Work out the finished part from the listing and answer in its coordinate system (mm). Round coordinates to 2 decimals unless told otherwise and drop trailing zeros. Write each loop counter-clockwise with the first axis right and the second up, starting at its lowest first coordinate (ties: lowest second). Pieces come first, ordered by that corner, then holes. Notation, with made-up numbers: (12, 50) -> (49, 50) arc R27 cw to (49, 81) -> close; hole circle Ø1 at (78, -7.5). An arc over 180 degrees is marked (long way). One line per item, written item: value.
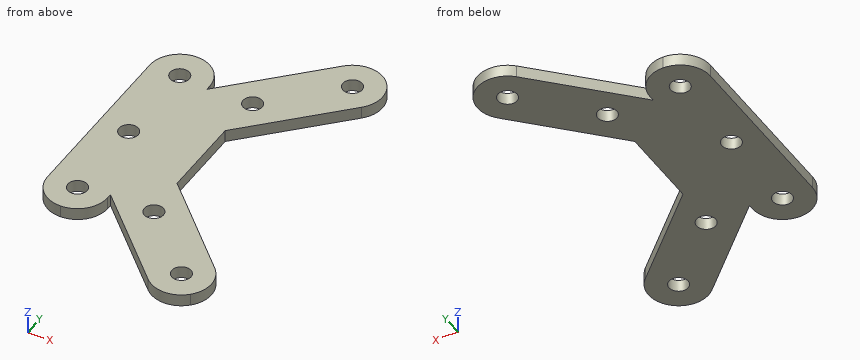
```python
from build123d import *

# Parameters (mm, degrees)
SKETCH_1_R          = 1.6
EXTRUDE_1_DEPTH     = 1
SKETCH_2_R          = 1.6
CUT_EXTRUDE_1_DEPTH = 45.10524807
FILLET_1_R          = 5


with BuildPart() as part:
    # ｽｹｯﾁ1 → ﾎﾞｽ - 押し出し1 (new, symmetric)
    with BuildSketch(Plane.XY):
        Polygon((5, 20), (-5, 20), (-5, -20), (5, -20), (5, -14.142135624), (23.03122292, -32.173358544), (30.102290732, -25.102290732), (12.071067812, -7.071067812), (12.071067812, 7.071067812), (30.102290732, 25.102290732), (23.03122292, 32.173358544), (5, 14.142135624), align=None)
        with Locations((0, -15)):
            Circle(SKETCH_1_R, mode=Mode.SUBTRACT)
        Circle(SKETCH_1_R, mode=Mode.SUBTRACT)
        with Locations((0, 15)):
            Circle(SKETCH_1_R, mode=Mode.SUBTRACT)
    extrude(amount=EXTRUDE_1_DEPTH, both=True)

    # ｽｹｯﾁ2 → ｶｯﾄ - 押し出し1 (cut, through all)
    with BuildSketch(Plane.XY.offset(1)):
        with Locations((12.424621202, 14.495689014)):
            Circle(SKETCH_2_R)
        with Locations((23.03122292, 25.102290732)):
            Circle(SKETCH_2_R)
        with Locations(Location((12.424621202, -14.495689014, 0), (0, 0, 180))):
            Circle(SKETCH_2_R)
        with Locations(Location((23.03122292, -25.102290732, 0), (0, 0, 180))):
            Circle(SKETCH_2_R)
    extrude(amount=-CUT_EXTRUDE_1_DEPTH, mode=Mode.SUBTRACT)

    # ﾌｨﾚｯﾄ1
    fillet_1_edges = [part.edges().sort_by_distance(p)[0] for p in [
        (5, -20, 0),
        (-5, -20, 0),
        (23.03122292, -32.173358544, 0),
        (30.102290732, -25.102290732, 0),
        (30.102290732, 25.102290732, 0),
        (23.03122292, 32.173358544, 0),
        (5, 20, 0),
        (-5, 20, 0),
    ]]
    fillet(fillet_1_edges, radius=FILLET_1_R - 0.0001)  # a hair under: the kernel refuses the full size


solid = part.part
```
(1) Flat-ended cylindrical pins translate along their axes: pin 1 Ø3 at (x, y) = (12.42, 14.5) entering from +Z; pin 2 Ø0.9 at (y, z) = (14.5, 0) entering from +X; pin 3 Ø1 at (y, z) = (-9.5, 0) entering from +X; pin 4 Ø1 at (y, z) = (-2.5, 0) entering from +X. Find the tip coordinate at first contact, or state that the pin passes through.
Reported:
pin 1: passes through
pin 2: stops at x = 19.95
pin 3: stops at x = 15
pin 4: stops at x = 12.07
(2) Find section C-C on y = -19. Give the vertices of the cut face in (x, z), plus the area to 3 significant figures.
Reported:
outline: (-3, -1) -> (3, -1) -> (3, 1) -> (-3, 1) -> close; (9.86, -1) -> (24, -1) -> (24, 1) -> (9.86, 1) -> close
area: 40.3 mm2
(3) Find section A-A on y = 0. Give the vertices of the cut face in (x, z).
Reported:
outline: (-5, -1) -> (-1.6, -1) -> (-1.6, 1) -> (-5, 1) -> close; (1.6, -1) -> (12.07, -1) -> (12.07, 1) -> (1.6, 1) -> close
(4) Find section B-B on z = -0.4. Give the number of separate pieces and of enclosed holes in the cut face, plus the area to 3 significant figures.
Reported:
separate pieces: 1
enclosed holes: 7
area: 961 mm2
(5) Consider probe 1 along Y at (x, z) = (0, 0.45); probe 2 along Y at (x, z) = (12.5, 0.3); probe 3 along Y at (x, z) = (11.5, -0.7). Determine where each line is inside the solid, lowest interval first.
Reported:
probe 1: y = -20 to -16.6, -13.4 to -1.6, 1.6 to 13.4, 16.6 to 20
probe 2: y = -21.64 to -16.09, -12.9 to -7.5, 7.5 to 12.9, 16.09 to 21.64
probe 3: y = -20.64 to -15.8, -13.19 to 13.19, 15.8 to 20.64
(6) Find section D-D on y = 8.5. Give the vertices of the cut face in (x, z).
Reported:
outline: (-5, -1) -> (13.5, -1) -> (13.5, 1) -> (-5, 1) -> close
